from build123d import *

# Parameters (mm, degrees)
SCHIZZO1_W                   = 27
SCHIZZO1_H                   = 32
ESTRUSIONE_ESTRUSIONE1_DEPTH = 31
SCHIZZO2_R                   = 1.5
TAGLIO_ESTRUSIONE1_DEPTH     = 32
SCHIZZO3_R                   = 4
TAGLIO_ESTRUSIONE2_DEPTH     = 33
SCHIZZO4_R                   = 5
TAGLIO_ESTRUSIONE5_DEPTH     = 1.5
SCHIZZO5_R                   = 5
TAGLIO_ESTRUSIONE6_DEPTH     = 1.5
SCHIZZO6_R                   = 2.5
TAGLIO_ESTRUSIONE7_DEPTH     = 15
SCHIZZO7_R                   = 2.5
TAGLIO_ESTRUSIONE8_DEPTH     = 10


with BuildPart() as part:
    # Schizzo1 → Estrusione-Estrusione1 (new body)
    with BuildSketch(Plane.XY):
        Rectangle(SCHIZZO1_W, SCHIZZO1_H)
    extrude(amount=ESTRUSIONE_ESTRUSIONE1_DEPTH)

    # Schizzo2 → Taglio-Estrusione1 (cut, through all)
    with BuildSketch(Plane(origin=(0, 0, 0), x_dir=(-1, 0, 0), z_dir=(0, 0, -1))):
        with Locations((-10, 10)):
            Circle(SCHIZZO2_R)
        with Locations((10, 10)):
            Circle(SCHIZZO2_R)
        with Locations((10, -10)):
            Circle(SCHIZZO2_R)
        with Locations((-10, -10)):
            Circle(SCHIZZO2_R)
    extrude(amount=-TAGLIO_ESTRUSIONE1_DEPTH, mode=Mode.SUBTRACT)

    # Schizzo3 → Taglio-Estrusione2 (cut, through all)
    with BuildSketch(Plane(origin=(0, 16, 0), x_dir=(1, 0, 0), z_dir=(0, 1, 0))):
        with Locations((0, -15.5)):
            Circle(SCHIZZO3_R)
    extrude(amount=-TAGLIO_ESTRUSIONE2_DEPTH, mode=Mode.SUBTRACT)

    # Schizzo4 → Taglio-Estrusione5 (cut)
    with BuildSketch(Plane(origin=(0, 16, 0), x_dir=(1, 0, 0), z_dir=(0, 1, 0))):
        with Locations((0, -15.5)):
            Circle(SCHIZZO4_R)
    extrude(amount=-TAGLIO_ESTRUSIONE5_DEPTH, mode=Mode.SUBTRACT)

    # Schizzo5 → Taglio-Estrusione6 (cut)
    with BuildSketch(Plane.XZ.offset(16)):
        with Locations((0, 15.5)):
            Circle(SCHIZZO5_R)
    extrude(amount=-TAGLIO_ESTRUSIONE6_DEPTH, mode=Mode.SUBTRACT)

    # Schizzo6 → Taglio-Estrusione7 (cut)
    with BuildSketch(Plane.XY.offset(31)):
        with Locations((-10, 10)):
            Circle(SCHIZZO6_R)
        with Locations((10, 10)):
            Circle(SCHIZZO6_R)
        with Locations((10, -10)):
            Circle(SCHIZZO6_R)
        with Locations((-10, -10)):
            Circle(SCHIZZO6_R)
    extrude(amount=-TAGLIO_ESTRUSIONE7_DEPTH, mode=Mode.SUBTRACT)

    # Schizzo7 → Taglio-Estrusione8 (cut)
    with BuildSketch(Plane.XY.offset(31)):
        with Locations((-5.5, 6)):
            Circle(SCHIZZO7_R)
        with Locations((5.5, 6)):
            Circle(SCHIZZO7_R)
        Circle(SCHIZZO7_R)
        with Locations((5.5, -6)):
            Circle(SCHIZZO7_R)
        with Locations((-5.5, -6)):
            Circle(SCHIZZO7_R)
    extrude(amount=-TAGLIO_ESTRUSIONE8_DEPTH, mode=Mode.SUBTRACT)


solid = part.part
Could you check a few things on this model? Use its own coordinates, in mm. A direction names the side the tool comes from. Coordinates: 2 decimals unless noted, no trailing zeros. Write each loop counter-clockwise with the first axis right and the second up, starting at its lowest first coordinate (ties: lowest second). Pieces come first, ordered by that corner, then holes. Notation, with made-up numbers: M -35,-10.75 L -15,-10.75 A25 cw -15,5.25 Z; hole C -2.75,-13.75 d2. An arc over 180 degrees is marked long. One line per question, with ' | ' between items.
1) I need wall thicknesses on probe 1 along Y at (x, z) = (10, 7.75); probe 2 along Y at (x, z) = (-10, 21.5); probe 3 along X at (y, z) = (6.75, 15.5). Which ranges of each line are inside material? Lowest first, please. Write a range as [from, to].
Checks:
probe 1: [-16, -11.5], [-8.5, 8.5], [11.5, 16] | probe 2: [-16, -12.5], [-7.5, 7.5], [12.5, 16] | probe 3: [-13.5, -4], [4, 13.5]
2) For pin 1 Ø2.5 at (x, y) = (-10, -10) entering from +Z; pin 2 Ø4 at (x, y) = (-10, 10) entering from +Z; pin 3 Ø3 at (x, z) = (2.5, 13.5) entering from +Y, each with a flat end and sliding along its axis, tell me the tip position at first contact or that it passes through.
Checks:
pin 1: through | pin 2: z = 16 | pin 3: y = 14.5
3) Imagine slicing it at C-C, the plane y = 6. Write out the boundary of the cut face in (x, z), and give its area (3 significant figures).
Checks:
outline: M -13.5,0 L 13.5,0 L 13.5,31 L 8,31 L 8,21 L 3,21 L 3,31 L -3,31 L -3,21 L -8,21 L -8,31 L -13.5,31 Z; hole C 0,15.5 d8 | area: 687 mm²
4) Imagine slicing it at A-A, the plane z = 15.5. Write out the boundary of the cut face in (x, y), and give its area (3 significant figures).
Checks:
outline: M -13.5,-16 L -5,-16 L -5,-14.5 L -4,-14.5 L -4,14.5 L -5,14.5 L -5,16 L -13.5,16 Z; M 4,-14.5 L 5,-14.5 L 5,-16 L 13.5,-16 L 13.5,16 L 5,16 L 5,14.5 L 4,14.5 Z; hole C -10,-10 d3; hole C -10,10 d3; hole C 10,-10 d3; hole C 10,10 d3 | area: 574 mm²
5) If we mould it in two halves opening along Y, with no side actions, what happens to faces 4 (the face through (13.5, 0, 15)), 5 (the face through (-6, 6, 21)), 6 (the face through (-4, 14.5, 17))? For each: released by +Y, released by -Y, zero draft, split by the parting line, or undercut.
Checks:
face 4: zero draft | face 5: undercut | face 6: released by +Y
6) For faces 1 (the face through (7.885, 6.751, 26.07)), 2 (the face through (-4, -14.5, 14)), 3 (the face through (3, 0, 31)), which set-ups out of +Z, -Z, +X, -X, +Y, -Y let a thin tool reach every point of the face, with its end or its side?
Checks:
face 1: +Z | face 2: -Y | face 3: +Z, +X, -X, +Y, -Y
7) Imagine slicing it at D-D, the plane z = 24.5. Give the number of separate pieces and of enclosed holes in the cut face, and give its area (3 significant figures).
Checks:
separate pieces: 1 | enclosed holes: 9 | area: 687 mm²
8) Imagine slicing it at B-B, the plane x = -10. Write out the boundary of the cut face in (y, z), and give its area (3 significant figures).
Checks:
outline: M -16,0 L -11.5,0 L -11.5,16 L -12.5,16 L -12.5,31 L -16,31 Z; M -8.5,0 L 8.5,0 L 8.5,16 L 7.5,16 L 7.5,31 L -7.5,31 L -7.5,16 L -8.5,16 Z; M 11.5,0 L 16,0 L 16,31 L 12.5,31 L 12.5,16 L 11.5,16 Z | area: 746 mm²
